```python
from build123d import *
from OCP.BRepFilletAPI import BRepFilletAPI_MakeChamfer

# Parameters (mm, degrees)
BOSS_EXTRUDE1_DEPTH = 20
SKETCH2_W           = 641.5
SKETCH2_H           = 23
SKETCH2_W_2         = 611.1
SKETCH2_H_2         = 8.73125
BOSS_EXTRUDE2_DEPTH = 6.35
SKETCH4_W           = 80
SKETCH4_H           = 19.05
BOSS_EXTRUDE3_DEPTH = 40
CUT_EXTRUDE2_DEPTH  = 50.8
CHAMFER1_SIZE       = 20
CHAMFER1_SIZE_2     = 3.526539614
FILLET1_R           = 10


with BuildPart() as part:
    # Sketch1 → Boss-Extrude1 (new body)
    with BuildSketch(Plane(origin=(0, 0, 0), x_dir=(1, 0, 0), z_dir=(0, 1, 0))):
        Polygon((-341.35, 23), (-341.35, 7.291), (-320.75, 7.291), (-320.75, -7.291), (-341.35, -7.291), (-341.35, -23), (341.35, -23), (341.35, -7.291), (320.75, -7.291), (320.75, 7.291), (341.35, 7.291), (341.35, 23), align=None)
    extrude(amount=BOSS_EXTRUDE1_DEPTH)

    # Sketch2 → Boss-Extrude2 (add)
    with BuildSketch(Plane(origin=(0, 20, 0), x_dir=(1, 0, 0), z_dir=(0, 1, 0))):
        with Locations((0, -11.5)):
            Rectangle(SKETCH2_W, SKETCH2_H)
        with Locations((0, -12.284375)):
            Rectangle(SKETCH2_W_2, SKETCH2_H_2, mode=Mode.SUBTRACT)
    extrude(amount=BOSS_EXTRUDE2_DEPTH)

    # Sketch4 → Boss-Extrude3 (add)
    with BuildSketch(Plane(origin=(0, 20, 0), x_dir=(1, 0, 0), z_dir=(0, 1, 0))):
        with Locations((0, 13.475)):
            Rectangle(SKETCH4_W, SKETCH4_H)
    extrude(amount=BOSS_EXTRUDE3_DEPTH)

    # Sketch5 → Cut-Extrude2 (cut)
    with BuildSketch(Plane(origin=(0, 0, -23), x_dir=(-1, 0, 0), z_dir=(0, 0, -1))):
        with BuildLine():
            ThreePointArc((3.407767598, 41.703883799), (0, 43.81), (-3.407767598, 41.703883799))
            Line((-3.407767598, 41.703883799), (0, 40))
            Line((0, 40), (3.407767598, 41.703883799))
        make_face()
        with BuildLine():
            Line((0, 40), (-3.407767598, 41.703883799))
            ThreePointArc((-3.407767598, 41.703883799), (-3.81, 40), (-3.407767598, 38.296116201))
            Line((-3.407767598, 38.296116201), (0, 40))
        make_face()
        with BuildLine():
            Line((3.407767598, 41.703883799), (0, 40))
            Line((0, 40), (3.407767598, 38.296116201))
            ThreePointArc((3.407767598, 38.296116201), (3.70807865, 39.124641373), (3.81, 40))
            ThreePointArc((3.81, 40), (3.70807865, 40.875358627), (3.407767598, 41.703883799))
        make_face()
        with BuildLine():
            Line((3.407767598, 38.296116201), (0, 40))
            Line((0, 40), (-3.407767598, 38.296116201))
            ThreePointArc((-3.407767598, 38.296116201), (0, 36.19), (3.407767598, 38.296116201))
        make_face()
    extrude(amount=-CUT_EXTRUDE2_DEPTH, mode=Mode.SUBTRACT)

    # Chamfer1
    chamfer1_edges_1 = [part.edges().sort_by_distance(p)[0] for p in [
        (331.05, 0, -7.291),
    ]]
    chamfer1_side_1 = [part.faces().sort_by_distance(p)[0] for p in [
        (331.05, 0.070530792, -7.291),
    ]]
    chamfer1_edges_2 = [part.edges().sort_by_distance(p)[0] for p in [
        (331.05, 0, 7.291),
    ]]
    chamfer1_side_2 = [part.faces().sort_by_distance(p)[0] for p in [
        (331.05, 0, 7.361530792),
    ]]
    chamfer1_edges_3 = [part.edges().sort_by_distance(p)[0] for p in [
        (-331.05, 0, 7.291),
    ]]
    chamfer1_side_3 = [part.faces().sort_by_distance(p)[0] for p in [
        (-331.05, 0, 7.361530792),
    ]]
    chamfer1_edges_4 = [part.edges().sort_by_distance(p)[0] for p in [
        (-331.05, 0, -7.291),
    ]]
    chamfer1_side_4 = [part.faces().sort_by_distance(p)[0] for p in [
        (-331.05, 0, -7.361530792),
    ]]
    chamfer1 = BRepFilletAPI_MakeChamfer(part.part.solid().wrapped)
    for e in chamfer1_edges_1:
        chamfer1.Add(CHAMFER1_SIZE - 0.0001, CHAMFER1_SIZE_2 - 0.0001, e.wrapped, chamfer1_side_1[0].wrapped)
    for e in chamfer1_edges_2:
        chamfer1.Add(CHAMFER1_SIZE_2 - 0.0001, CHAMFER1_SIZE - 0.0001, e.wrapped, chamfer1_side_2[0].wrapped)
    for e in chamfer1_edges_3:
        chamfer1.Add(CHAMFER1_SIZE_2 - 0.0001, CHAMFER1_SIZE - 0.0001, e.wrapped, chamfer1_side_3[0].wrapped)
    for e in chamfer1_edges_4:
        chamfer1.Add(CHAMFER1_SIZE_2 - 0.0001, CHAMFER1_SIZE - 0.0001, e.wrapped, chamfer1_side_4[0].wrapped)
    add(Compound.cast(chamfer1.Shape()), mode=Mode.REPLACE)  # a hair under: the kernel refuses the full size

    # Fillet1
    fillet1_edges = [part.edges().sort_by_distance(p)[0] for p in [
        (40, 20, -13.475),
        (-40, 60, -13.475),
        (40, 60, -13.475),
        (-40, 20, -13.475),
    ]]
    fillet(fillet1_edges, radius=FILLET1_R)


solid = part.part
```
The model under review builds one solid part; all positions refer to its coordinate system, in mm. A direction names the side the tool comes from. Round coordinates to 2 decimals unless told otherwise and drop trailing zeros. Order: outer loops, then holes, each group sorted by start corner. A loop starts at its lowest first (then second) coordinate and runs counter-clockwise, first axis right, second up. Notation, with made-up numbers: (54.5, -5.75) -> (86.5, -5.75) arc R15 cw to (86.5, 8.25) -> close; hole circle Ø3 at (-29, -20.75). An arc over 180 degrees is marked (long way). One line per item, written item: value. Start each with the question number.
Q1. Take a section at B-B (y = 12). Write out the cut boundary in (x, z), and give its area (3 significant figures).
Q2. Machinability: for faces 1 (the face through (-330.91, 10.14, 9.03)), 2 (the face through (331, 20, 15)), 3 (the face through (-1, 35, -3.95)), 4 (the face through (330.91, 9.86, -9.08)), which of the approach directions +Z, -Z, +X, -X, +Y, -Y give a long, thin tool a straight path to every point of the face, cutting with its end or side? Answer none if there is none.
Q3. Clearance check with flat-ended pins moving along their axes: pin 1 Ø17.5 at (x, z) = (-332, 14) entering from +Y; pin 2 Ø7 at (x, z) = (160, 13.5) entering from +Y; pin 3 Ø5.5 at (y, z) = (44, -10) entering from +X. State where each tip first meets the part, or that it passes through.
Q4. Take a section at A-A (z = -17.5). Write out the cut boundary in (x, y).
Q5. Mouldability with a two-part tool opening along Z and no side actions: class faces 5 (the face through (-331.19, 10.14, -9.03)), 6 (the face through (40, 40, -13)), 7 (the face through (5, 16, -23)) as released by +Z, released by -Z, zero draft, split by the parting line, or undercut.
Q6. Take a section at C-C (x = -169.5). Write out the cut boundary in (y, z), and give its area (3 significant figures).
Q7. Wall thickness on line 1 (Z direction, x = 34, y = 23); line 2 (Z direction, x = 58, y = 21.5); line 3 (Z direction, x = -5.5, y = 28.5): over which ranges is each line inside the solid? List them lowest first.
Reported:
1. outline: (-341.35, -23) -> (341.35, -23) -> (341.35, -8.7) -> (320.75, -8.7) -> (320.75, 8.7) -> (341.35, 8.7) -> (341.35, 23) -> (-341.35, 23) -> (-341.35, 8.7) -> (-320.75, 8.7) -> (-320.75, -8.7) -> (-341.35, -8.7) -> close
1. area: 30,700 mm2
2. face 1: -X, -Y
2. face 2: +Z, -Z, +X, +Y
2. face 3: +X, -X, +Y
2. face 4: +X, -Y
3. pin 1: stops at y = 20
3. pin 2: stops at y = 26.35
3. pin 3: stops at x = 40
4. outline: (-341.35, 0) -> (341.35, 0) -> (341.35, 20) -> (50, 20) arc R10 cw to (40, 30) -> (40, 50) arc R10 ccw to (30, 60) -> (-30, 60) arc R10 ccw to (-40, 50) -> (-40, 30) arc R10 cw to (-50, 20) -> (-341.35, 20) -> close; hole circle Ø7.62 at (0, 40)
5. face 5: undercut
5. face 6: zero draft
5. face 7: released by -Z
6. outline: (0, -23) -> (20, -23) -> (20, 0) -> (26.35, 0) -> (26.35, 7.92) -> (20, 7.92) -> (20, 16.65) -> (26.35, 16.65) -> (26.35, 23) -> (0, 23) -> close
6. area: 1,010 mm2
7. line 1: z = -23 to -3.95, 0 to 7.92, 16.65 to 23
7. line 2: z = 0 to 7.92, 16.65 to 23
7. line 3: z = -23 to -3.95
